Autodesk Inventor part; units mm, degrees
ref_plane "YZ Plane" through (0, 0, 0) normal (1, 0, 0) x (0, 1, 0)
ref_plane "XZ Plane" through (0, 0, 0) normal (0, 1, 0) x (-1, 0, 0)
ref_plane "XY Plane" through (0, 0, 0) normal (0, 0, 1) x (1, 0, 0)
sketch "Sketch1" plane through (0, 0, 0) normal (0, 1, 0) x (-1, 0, 0)
  circle A0 centre (0, 0) radius 25.4
  dimension "d0" = 50.8
extrude "Extrusion1" add sketch "Sketch1" along normal blind 3.175
sketch "Sketch2" plane through (0, 3.175, 0) normal (0, 1, 0) x (1, 0, 0)
  circle A0 centre (0, 0) radius 25.4
  circle A1 centre (0, 0) radius 22.225
  dimension "d3" = 3.175
  dimension "d4" = 50.8
extrude "Extrusion2" add sketch "Sketch2" along normal blind 292.1
sketch "Sketch3" plane through (0, 295.275, 0) normal (0, 1, 0) x (1, 0, 0)
  circle A0 centre (0, 0) radius 25.4
extrude "Extrusion3" add sketch "Sketch3" along normal blind 3.175
sketch "Sketch4" plane through (0, 298.45, 0) normal (0, 1, 0) x (1, 0, 0)
  line L0 (0, 7.3323) -> (6.35, 3.6662)
  line L1 (6.35, 3.6662) -> (6.35, -3.6662)
  line L2 (6.35, -3.6662) -> (0, -7.3323)
  line L3 (0, -7.3323) -> (-6.35, -3.6662)
  line L4 (-6.35, -3.6662) -> (-6.35, 3.6662)
  line L5 (-6.35, 3.6662) -> (0, 7.3323)
  point P0 (0, 0)
  point P1 (0, 0)
  dimension "d9" = 12.7
extrude "Extrusion4" cut sketch "Sketch4" against normal through all
Could you check a few things on this model? Use its own coordinates, in mm. A direction names the side the tool comes from. Round coordinates to 2 decimals unless told otherwise and drop trailing zeros. Loops run counter-clockwise (first coordinate to the right, second up) from the corner with the lowest first, then second, coordinate; pieces in that order, holes last. Notation, with made-up numbers: (22.25, -6.75) - (53.25, -6.75) arc R17 ccw to (53.25, 13.25) - close; hole circle Ø4 at (43.5, 78). An arc over 180 degrees is marked (long way). Write item = value, one per line.
1) I need wall thicknesses on line 1 along Y through (x, z) = (-15.5, -8.5) (3 decimals); line 2 along Z through (x, y) = (0, 171) (3 decimals). Which ranges of each line are inside material? Lowest first, please. Write a range as from..to.
Computed:
line_1 = 0..3.175, 295.275..298.45
line_2 = -25.4..-22.225, 22.225..25.4
2) If we mould it in two halves opening along Z, with no side actions, what happens to faces 1 (the flat face through (5, 3.175, -5)), 2 (the flat face through (5, 298.45, 5))? For each: pulls with the +Z half, pulls with the -Z half, needs draft (parallel to the pull), parting line crosses it, or undercut.
Computed:
face_1 = undercut
face_2 = needs draft
3) I'm going to push flat-ended pins straight in: P1, Ø6, axis at x = 11.5, y = 88, coming from the +Z side; P2, Ø4, axis at y = 151, z = 17.5, coming from the +X side; P3, Ø6, axis at y = 145.5, z = -17, coming from the +X side; P4, Ø22, axis at x = 3.5, z = 1.5, coming from the +Y side. Where does each tip first touch, or does it pass through?
Computed:
P1 = 23.94
P2 = 20.12
P3 = 21.19
P4 = 298.45
4) Imagine slicing it at A-A (y = 84). Please give me the cut outline in (x, z) (3 decimals).
Computed:
outline = circle Ø50.8 at (0, 0); hole circle Ø44.45 at (0, 0)
5) On a 3-axis mill with a long thin cutter (end or side, diameter ignored), from which of +Z, -Z, +X, -X, +Y, -Y can I reach the whole of each face in a straight line? I mean faces 3 (the cylindrical face through (21.199, 147.18, 6.676)), 4 (the flat face through (-5, 0, -5)). Say none if no direction works.
Computed:
face_3 = none
face_4 = +Z, -Z, +X, -X, -Y
